from build123d import *

# Parameters (mm, degrees)
BOSS_EXTRUDE1_DEPTH = 2
FILLET1_R           = 0.5
SKETCH2_R           = 2
CUT_EXTRUDE1_DEPTH  = 2


with BuildPart() as part:
    # Sketch1 → Boss-Extrude1 (new body)
    with BuildSketch(Plane.YZ):
        Polygon((0, 0), (8, 0), (8, 7), (6, 7), (6, 34.5), (-6, 34.5), (-6, 7), (-8, 7), (-8, 0), align=None)
    extrude(amount=BOSS_EXTRUDE1_DEPTH)

    # Fillet1
    fillet1_edges = [part.edges().sort_by_distance(p)[0] for p in [
        (1, 6, 34.5),
        (1, 8, 0),
        (1, -8, 0),
        (1, -6, 34.5),
    ]]
    fillet(fillet1_edges, radius=FILLET1_R)

    # Sketch2 → Cut-Extrude1 (cut)
    with BuildSketch(Plane.YZ.offset(2)):
        with Locations(Location((0, 29, 0), (0, 0, 270))):
            Circle(SKETCH2_R)
        with BuildLine():
            Line((-2, 12.5), (-2, 10.5))
            ThreePointArc((-2, 10.5), (0, 8.5), (2, 10.5))
            Line((2, 10.5), (2, 12.5))
            ThreePointArc((2, 12.5), (0, 14.5), (-2, 12.5))
        make_face()
    extrude(amount=-CUT_EXTRUDE1_DEPTH, mode=Mode.SUBTRACT)


solid = part.part
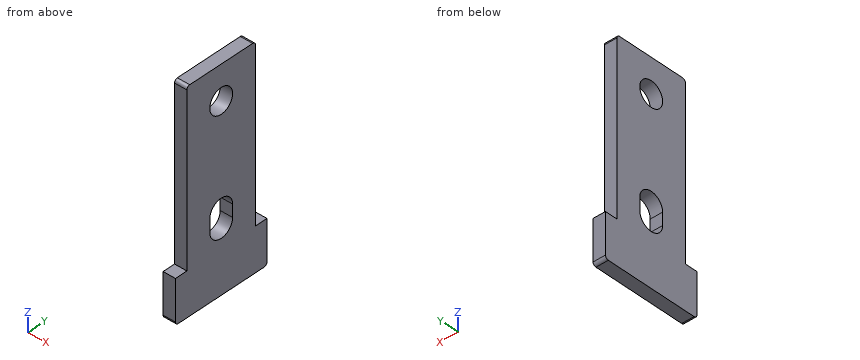
For this review, take the finished solid that the model builds, in its own axes (mm). Round coordinates to 2 decimals unless told otherwise and drop trailing zeros. Write each loop counter-clockwise with the first axis right and the second up, starting at its lowest first coordinate (ties: lowest second). Pieces come first, ordered by that corner, then holes. Notation, with made-up numbers: (37.25, 29.25) - (66.25, 29.25) arc R14 cw to (66.25, 38.25) - close; hole circle Ø3 at (-24.5, 45). An arc over 180 degrees is marked (long way). Write item = value, one per line. Start each with the question number.
1. Wall thickness on L1, parallel to Y at x = 1.2, z = 29; L2, parallel to Z at x = 1.35, y = 0.25; L3, parallel to Y at x = 1, z = 25: over which ranges is each line inside the solid? List them lowest first.
2. Consider section B-B on x = 1. State the section outline as (y, z) points.
3. Consider section A-A on y = 0. State the section outline as (x, z) points.
4. For pin 1 Ø1.5 at (y, z) = (-5.5, 18) entering from -X; pin 2 Ø0.6 at (x, y) = (1, 7) entering from +Z; pin 3 Ø0.6 at (x, z) = (0.5, 11) entering from +Y, all flat-tipped, find the tip position at first contact; note any pin that passes through.
5. Consider section C-C on z = 29. State the section outline as (x, y) points, plus the area to 3 significant figures.
Evaluation:
q1.L1 = -6 to -2, 2 to 6
q1.L2 = 0 to 8.52, 14.48 to 27.02, 30.98 to 34.5
q1.L3 = -6 to 6
q2.outline = (-8, 0.5) arc R0.5 ccw to (-7.5, 0) - (7.5, 0) arc R0.5 ccw to (8, 0.5) - (8, 7) - (6, 7) - (6, 34) arc R0.5 ccw to (5.5, 34.5) - (-5.5, 34.5) arc R0.5 ccw to (-6, 34) - (-6, 7) - (-8, 7) - close; hole (-2, 10.5) arc R2 ccw to (2, 10.5) - (2, 12.5) arc R2 ccw to (-2, 12.5) - close; hole circle Ø4 at (0, 29)
q3.outline = (0, 0) - (2, 0) - (2, 8.5) - (0, 8.5) - close; (0, 14.5) - (2, 14.5) - (2, 27) - (0, 27) - close; (0, 31) - (2, 31) - (2, 34.5) - (0, 34.5) - close
q4.pin_1 = 0
q4.pin_2 = 7
q4.pin_3 = 6
q5.outline = (0, -6) - (2, -6) - (2, -2) - (0, -2) - close; (0, 2) - (2, 2) - (2, 6) - (0, 6) - close
q5.area = 16.0 mm2
